Read the model definition and answer for the solid it produces. Units are mm, in the model's axes. A direction names the side the tool comes from. Coordinates: 2 decimals unless noted, no trailing zeros. Loops run counter-clockwise (first coordinate to the right, second up) from the corner with the lowest first, then second, coordinate; pieces in that order, holes last. Notation, with made-up numbers: M -9,-2.75 L 4,-2.75 A27 ccw 4,17.25 Z; hole C -6.5,-8.75 d8. An arc over 180 degrees is marked long. Use one line per item in the form item = value. Start each with the question number.
1. Flat-ended cylindrical pins translate along their axes: pin 1 (1 mm diameter, centred on y = 2, z = 14.5, fed in from +X) (3 decimals); pin 2 (5 mm diameter, centred on x = -1.43, y = -1.69, fed in from -Z); pin 3 (0.6 mm diameter, centred on x = 3.5, z = -1.5, fed in from -Y); pin 4 (0.6 mm diameter, centred on y = 2.5, z = -2.5, fed in from -X) (3 decimals). Find the tip coordinate at first contact, or state that the pin passes through.
2. The part is cut by section C-C (y = 4.5). Give the vertices of the cut face in (x, z) (3 decimals), plus the area to 3 significant figures.
3. A tool of negligible diameter and unlimited length cuts with its end or side. For faces 4 (the flat face through (-1.135, 2, 15)), 5 (the flat face through (2, 4.15, 15)), 6 (the flat face through (-2, 0.65, 15)), 7 (the cylindrical face through (3.816, -1.235, 11.053)), from which of +Z, -Z, +X, -X, +Y, -Y can it reach the whole face along a straight path? Write none if from no direction.
4. Find the intervals of material crossed by probe 1 along X at (y, z) = (2.5, 15.25) (3 decimals); probe 2 along Z at (x, y) = (4, 4.5); probe 3 along Z at (x, y) = (1.25, -1.5), in increasing order. Write a range as [from, to].
5. The part is cut by section B-B (y = 1.25). Give the vertices of the cut face in (x, z) (3 decimals).
6. For a pull along X with two mould halves and no side action, classify faces 1 (the cylindrical face through (0.006, -1.235, 11.053)), 2 (the flat face through (2.675, 2, 15)), 3 (the flat face through (-2, 4.15, 15)) as released by +X, released by -X, zero draft, split by the parting line, or undercut.
7. The part is cut by section D-D (y = -1.25). Give the vertices of the cut face in (x, z) (3 decimals), plus the area to 3 significant figures.
8. The part is cut by section A-A (z = 13.25). Give the vertices of the cut face in (x, y) (3 decimals).
from build123d import *
from OCP.BRepFilletAPI import BRepFilletAPI_MakeChamfer

# Parameters (mm, degrees)
SKETCH_1_W                          = 8.97
SKETCH_1_H                          = 10.8
EXTRUDE_1_DEPTH                     = 13
FILLET_1_SIZE                       = 1
FILLET_1_SIZE_2                     = 1.5
SKETCH_2_W                          = 2
SKETCH_2_H                          = 3.5
EXTRUDE_2_DEPTH                     = 3.95
SKETCH_3_R                          = 1.5
CUT_EXTRUDE_1_DEPTH                 = 3.95
SKETCH_4_W                          = 0.5
SKETCH_4_H                          = 0.8
EXTRUDE_3_DEPTH                     = 3.5
CHAMFER_1_SIZE                      = 0.5
CHAMFER_1_SIZE2                     = 0.288675135
PATTERN_LINEAR_2_COUNT              = 2
PATTERN_LINEAR_2_PITCH              = 3.81
CHAMFER_1_OF_PATTERN_LINEAR_2_SIZE  = 0.5
CHAMFER_1_OF_PATTERN_LINEAR_2_SIZE2 = 0.288675135


with BuildPart() as part:
    # Эскиз1 → Бобышка-Вытянуть1 (new body)
    with BuildSketch(Plane.XY):
        Rectangle(SKETCH_1_W, SKETCH_1_H)
    extrude(amount=EXTRUDE_1_DEPTH)

    # Скругление1
    # an asymmetric fillet: 1.5, 1 mm, written as the material it takes off along each edge
    with BuildSketch(Plane(origin=(-8.235, -5.4, 13), x_dir=(0, 0, -1), z_dir=(1, 0, 0))) as fillet_1_piece_1:
        with BuildLine():
            Bezier((FILLET_1_SIZE, 0), (0, 0), (0, FILLET_1_SIZE_2), weights=[1, 0.707106781, 1])
            Line((0, FILLET_1_SIZE_2), (0, 0))
            Line((0, 0), (FILLET_1_SIZE, 0))
        make_face()
    extrude(amount=16.47, mode=Mode.SUBTRACT)

    # Эскиз2 → Бобышка-Вытянуть2 (add)
    with BuildSketch(Plane.XY.offset(13)):
        with Locations((1.675, 2.4)):
            Rectangle(SKETCH_2_W, SKETCH_2_H)
    extrude_2 = extrude(amount=EXTRUDE_2_DEPTH)

    # Эскиз3 → Вырез-Вытянуть1 (cut)
    with BuildSketch(Plane.XY.offset(13)):
        with Locations((2.385, -1.686021073)):
            Circle(SKETCH_3_R)
    cut_extrude_1 = extrude(amount=-CUT_EXTRUDE_1_DEPTH, mode=Mode.SUBTRACT)

    # Эскиз4 → Бобышка-Вытянуть3 (add)
    with BuildSketch(Plane(origin=(0, 0, 0), x_dir=(-1, 0, 0), z_dir=(0, 0, -1))):
        with Locations((-3.445, 2.85)):
            Rectangle(SKETCH_4_W, SKETCH_4_H)
        with Locations((-3.445, -2.15)):
            Rectangle(SKETCH_4_W, SKETCH_4_H)
    extrude_3 = extrude(amount=EXTRUDE_3_DEPTH)

    # Фаска1: one chamfer whose edges measure the first distance from different faces: ONE call of the kernel's chamfer builder (chamfer() names one face for all edges)
    chamfer_1_edges_1 = [part.edges().sort_by_distance(p)[0] for p in [
        (3.445, 3.25, -3.5),
    ]]
    chamfer_1_side_1 = [part.faces().sort_by_distance(p)[0] for p in [
        (3.445, 3.25, -1.75),
    ]]
    chamfer_1_edges_2 = [part.edges().sort_by_distance(p)[0] for p in [
        (3.445, 2.45, -3.5),
    ]]
    chamfer_1_side_2 = [part.faces().sort_by_distance(p)[0] for p in [
        (3.445, 2.45, -1.75),
    ]]
    chamfer_1_edges_3 = [part.edges().sort_by_distance(p)[0] for p in [
        (3.445, -2.55, -3.5),
    ]]
    chamfer_1_side_3 = [part.faces().sort_by_distance(p)[0] for p in [
        (3.445, -2.55, -1.75),
    ]]
    chamfer_1_edges_4 = [part.edges().sort_by_distance(p)[0] for p in [
        (3.445, -1.75, -3.5),
    ]]
    chamfer_1_side_4 = [part.faces().sort_by_distance(p)[0] for p in [
        (3.445, -1.75, -1.75),
    ]]
    chamfer_1 = BRepFilletAPI_MakeChamfer(part.part.solid().wrapped)
    for e in chamfer_1_edges_1:
        chamfer_1.Add(CHAMFER_1_SIZE, CHAMFER_1_SIZE2, e.wrapped, chamfer_1_side_1[0].wrapped)  # the first distance lies on this face
    for e in chamfer_1_edges_2:
        chamfer_1.Add(CHAMFER_1_SIZE, CHAMFER_1_SIZE2, e.wrapped, chamfer_1_side_2[0].wrapped)  # the first distance lies on this face
    for e in chamfer_1_edges_3:
        chamfer_1.Add(CHAMFER_1_SIZE, CHAMFER_1_SIZE2, e.wrapped, chamfer_1_side_3[0].wrapped)  # the first distance lies on this face
    for e in chamfer_1_edges_4:
        chamfer_1.Add(CHAMFER_1_SIZE, CHAMFER_1_SIZE2, e.wrapped, chamfer_1_side_4[0].wrapped)  # the first distance lies on this face
    add(Compound.cast(chamfer_1.Shape()), mode=Mode.REPLACE)

    # Линейный массив2: Бобышка-Вытянуть2, Вырез-Вытянуть1, Бобышка-Вытянуть3 ×2
    with Locations(*[(-i * PATTERN_LINEAR_2_PITCH, 0, 0) for i in range(1, PATTERN_LINEAR_2_COUNT)]):
        add(extrude_2)
        add(cut_extrude_1, mode=Mode.SUBTRACT)
        add(extrude_3)

    # Фаска1 of Линейный массив2: one chamfer whose edges measure the first distance from different faces: ONE call of the kernel's chamfer builder (chamfer() names one face for all edges)
    chamfer_1_of_pattern_linear_2_edges_1 = [part.edges().sort_by_distance(p)[0] for p in [
        (-0.365, 3.25, -3.5),
    ]]
    chamfer_1_of_pattern_linear_2_side_1 = [part.faces().sort_by_distance(p)[0] for p in [
        (-0.365, 3.25, -1.75),
    ]]
    chamfer_1_of_pattern_linear_2_edges_2 = [part.edges().sort_by_distance(p)[0] for p in [
        (-0.365, 2.45, -3.5),
    ]]
    chamfer_1_of_pattern_linear_2_side_2 = [part.faces().sort_by_distance(p)[0] for p in [
        (-0.365, 2.45, -1.75),
    ]]
    chamfer_1_of_pattern_linear_2_edges_3 = [part.edges().sort_by_distance(p)[0] for p in [
        (-0.365, -2.55, -3.5),
    ]]
    chamfer_1_of_pattern_linear_2_side_3 = [part.faces().sort_by_distance(p)[0] for p in [
        (-0.365, -2.55, -1.75),
    ]]
    chamfer_1_of_pattern_linear_2_edges_4 = [part.edges().sort_by_distance(p)[0] for p in [
        (-0.365, -1.75, -3.5),
    ]]
    chamfer_1_of_pattern_linear_2_side_4 = [part.faces().sort_by_distance(p)[0] for p in [
        (-0.365, -1.75, -1.75),
    ]]
    chamfer_1_of_pattern_linear_2 = BRepFilletAPI_MakeChamfer(part.part.solid().wrapped)
    for e in chamfer_1_of_pattern_linear_2_edges_1:
        chamfer_1_of_pattern_linear_2.Add(CHAMFER_1_OF_PATTERN_LINEAR_2_SIZE, CHAMFER_1_OF_PATTERN_LINEAR_2_SIZE2, e.wrapped, chamfer_1_of_pattern_linear_2_side_1[0].wrapped)  # the first distance lies on this face
    for e in chamfer_1_of_pattern_linear_2_edges_2:
        chamfer_1_of_pattern_linear_2.Add(CHAMFER_1_OF_PATTERN_LINEAR_2_SIZE, CHAMFER_1_OF_PATTERN_LINEAR_2_SIZE2, e.wrapped, chamfer_1_of_pattern_linear_2_side_2[0].wrapped)  # the first distance lies on this face
    for e in chamfer_1_of_pattern_linear_2_edges_3:
        chamfer_1_of_pattern_linear_2.Add(CHAMFER_1_OF_PATTERN_LINEAR_2_SIZE, CHAMFER_1_OF_PATTERN_LINEAR_2_SIZE2, e.wrapped, chamfer_1_of_pattern_linear_2_side_3[0].wrapped)  # the first distance lies on this face
    for e in chamfer_1_of_pattern_linear_2_edges_4:
        chamfer_1_of_pattern_linear_2.Add(CHAMFER_1_OF_PATTERN_LINEAR_2_SIZE, CHAMFER_1_OF_PATTERN_LINEAR_2_SIZE2, e.wrapped, chamfer_1_of_pattern_linear_2_side_4[0].wrapped)  # the first distance lies on this face
    add(Compound.cast(chamfer_1_of_pattern_linear_2.Shape()), mode=Mode.REPLACE)


solid = part.part
Computed values:
q1.pin_1 = 2.675
q1.pin_2 = -3.5
q1.pin_3 = -2.55
q1.pin_4 = -0.615
q2.outline = M -4.485,0 L 4.485,0 L 4.485,13 L -4.485,13 Z
q2.area = 117 mm²
q3.face_4 = +Z, +Y, -Y
q3.face_5 = +Z, +X, -X, +Y
q3.face_6 = +Z, +X, -X, -Y
q3.face_7 = +Z
q4.probe_1 = [-3.135, -1.135], [0.675, 2.675]
q4.probe_2 = [0, 13]
q4.probe_3 = [0, 9.05]
q5.outline = M -4.485,0 L 4.485,0 L 4.485,13 L 2.675,13 L 2.675,16.95 L 0.675,16.95 L 0.675,13 L -1.135,13 L -1.135,16.95 L -3.135,16.95 L -3.135,13 L -4.485,13 Z
q6.face_1 = undercut
q6.face_2 = released by +X
q6.face_3 = zero draft
q7.outline = M -4.485,0 L 4.485,0 L 4.485,13 L 3.82,13 L 3.82,9.05 L 0.95,9.05 L 0.95,13 L 0.01,13 L 0.01,9.05 L -2.86,9.05 L -2.86,13 L -4.485,13 Z
q7.area = 93.9 mm²
q8.outline = M -3.135,0.65 L -1.135,0.65 L -1.135,4.15 L -3.135,4.15 Z; M 0.675,0.65 L 2.675,0.65 L 2.675,4.15 L 0.675,4.15 Z
